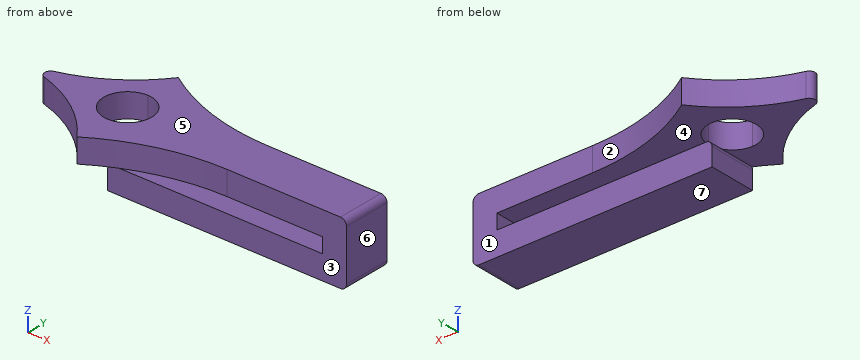
```python
from build123d import *

# Parameters (mm, degrees)
F4_DEPTH = 2
F5_DEPTH = 1.25
F6_START = -1.25
F6_DEPTH = 2
F8_DEPTH = 4


# Not quite as in the source:
# - a feature names something its author has since deleted; it is built from what else it names


with BuildPart() as f4:
    # F3 (on Top) → F4 (new body)
    with BuildSketch(Plane.XY):
        with BuildLine():
            Line((0, -2), (0, 0))
            Line((0, 0), (0, 2))
            Line((0, 2), (-8, 2))
            Line((-8, 2), (-18, 2))
            ThreePointArc((-18, 2), (-16.5857864376, 1.4142135624), (-16, 0))
            ThreePointArc((-16, 0), (-16.5857864376, -1.4142135624), (-18, -2))
            Line((-18, -2), (-8, -2))
            Line((-8, -2), (0, -2))
        make_face()
        Polygon((0, 2), (0, 0), (0, -2), (2, -2), (2, 2), align=None)
        with BuildLine():
            Line((-18, 2), (-8, 2))
            ThreePointArc((-8, 2), (-13.2201532545, 2.7661558185), (-18, 5))
            ThreePointArc((-18, 5), (-20.9134084444, 2.2029023447), (-24.5666209478, 0.4807692308))
            ThreePointArc((-24.5666209478, 0.4807692308), (-24.9292857857, 0), (-24.5666209478, -0.4807692308))
            ThreePointArc((-24.5666209478, -0.4807692308), (-20.9134084444, -2.2029023447), (-18, -5))
            ThreePointArc((-18, -5), (-13.2201532545, -2.7661558185), (-8, -2))
            Line((-8, -2), (-18, -2))
            ThreePointArc((-18, -2), (-20, 0), (-18, 2))
        make_face()
    extrude(amount=F4_DEPTH)

    # F3 (on Top) → F5 (join)
    with BuildSketch(Plane.XY):
        Polygon((0, 2), (0, 0), (0, -2), (2, -2), (2, 2), align=None)
    extrude(amount=-F5_DEPTH)

    # F3 (on Top) → F6 (join)
    with BuildSketch(Plane.XY.offset(F6_START)):
        with BuildLine():
            Line((0, -2), (0, 0))
            Line((0, 0), (0, 2))
            Line((0, 2), (-8, 2))
            Line((-8, 2), (-18, 2))
            ThreePointArc((-18, 2), (-16.5857864376, 1.4142135624), (-16, 0))
            ThreePointArc((-16, 0), (-16.5857864376, -1.4142135624), (-18, -2))
            Line((-18, -2), (-8, -2))
            Line((-8, -2), (0, -2))
        make_face()
        Polygon((0, 2), (0, 0), (0, -2), (2, -2), (2, 2), align=None)
        with BuildLine():
            ThreePointArc((-16, 0), (-16.5857864376, 1.4142135624), (-18, 2))
            Line((-18, 2), (-18, -2))
            ThreePointArc((-18, -2), (-16.5857864376, -1.4142135624), (-16, 0))
        make_face()
    extrude(amount=-F6_DEPTH)

    # F7 (on face) → F8 (cut)
    with BuildSketch(Plane.XZ.offset(2)):
        with BuildLine():
            Line((-18, -1.25), (-18, -1.75))
            ThreePointArc((-18, -1.75), (-17.8535533906, -1.3964466094), (-17.5, -1.25))
            Line((-17.5, -1.25), (-18, -1.25))
        make_face()
        with BuildLine():
            ThreePointArc((1.5, 2), (1.8535533906, 1.8535533906), (2, 1.5))
            Line((2, 1.5), (2, 2))
            Line((2, 2), (1.5, 2))
        make_face()
        with BuildLine():
            ThreePointArc((2, -2.75), (1.8535533906, -3.1035533906), (1.5, -3.25))
            Line((1.5, -3.25), (2, -3.25))
            Line((2, -3.25), (2, -2.75))
        make_face()
    extrude(amount=-F8_DEPTH, mode=Mode.SUBTRACT)


solid = f4.part
```
CAD build for the part. Positions are in the model's coordinates, mm. Face numbers are marked on the shaded views. A direction names the side the tool comes from. Round coordinates to 2 decimals unless told otherwise and drop trailing zeros. Loops run counter-clockwise (first coordinate to the right, second up) from the corner with the lowest first, then second, coordinate; pieces in that order, holes last. Notation, with made-up numbers: (9.5, 82) - (13.5, 82) arc R29 cw to (13.5, 102) - close; hole circle Ø1 at (24, 37.5). An arc over 180 degrees is marked (long way). Return JSON: item names as keys, results as strings. Group by question number.
Q1. Band-saw the part on D-D on z = -2.1. Give the cut face in (x, y), plus the area to 3 significant figures.
Q2. Band-saw the part on A-A on z = 0.9. Give the cut face in (x, y).
Q3. Two-plate mould, pull along Z, no slides. Class the marked faces 4, 5, 6 and 7: +Z half, -Z half, draft (parallel to the pull), parting line (faces both ways), or undercut.
Q4. Band-saw the part on C-C on x = -17. Give the cut face in (y, z).
Q5. Tool access for the marked faces 1, 2 and 3: list every direction of +Z, -Z, +X, -X, +Y, -Y with a clear straight run to the whole face (end or side of a thin tool).
Q6. Drill centre lines: line 1 along Z through (x, y) = (-6.5, 0.5); line 2 along Z through (x, y) = (-18.5, 4.25); line 3 along Y through (x, z) = (-2, 0.3). Where is each one in solid material? Low to high. Write a range as [from, to].
Q7. Band-saw the part on B-B on x = -9.5. Give the cut face in (y, z).
Q8. Flat gauge pins, fed straight in: pin 1 Ø2.5 at (x, z) = (-3.5, 0) entering from -Y; pin 2 Ø1.4 at (y, z) = (0, -0.5) entering from -X; pin 3 Ø0.8 at (y, z) = (0, -2.5) entering from -X. Where does each tip first touch, or does it go through?
Solutions:
{
 "1": {"outline": "(-18, -2) - (2, -2) - (2, 2) - (-18, 2) - close", "area": "80.0 mm^2"},
 "2": {"outline": "(-24.57, -0.48) arc R12.5 cw to (-18, -5) arc R18.17 cw to (-8, -2) - (2, -2) - (2, 2) - (-8, 2) arc R18.17 cw to (-18, 5) arc R12.5 cw to (-24.57, 0.48) arc R0.5 ccw to start; hole circle Ø4 at (-18, 0)"},
 "3": {"face 4": "undercut", "face 5": "+Z half", "face 6": "draft", "face 7": "-Z half"},
 "4": {"outline": "(-4.39, 0) - (-1.73, 0) - (-1.73, 2) - (-4.39, 2) - close; (-2, -3.25) - (2, -3.25) - (2, -1.25) - (-2, -1.25) - close; (1.73, 0) - (4.39, 0) - (4.39, 2) - (1.73, 2) - close"},
 "5": {"face 1": "-Z, +X, +Y", "face 2": "+Z, -Z, +X, +Y", "face 3": "-Z, +X, -Y"},
 "6": {"line 1": "z = [-3.25, -1.25], [0, 2]", "line 2": "z = [0, 2]", "line 3": "y = [-2, 2]"},
 "7": {"outline": "(-2.06, 0) - (2.06, 0) - (2.06, 2) - (-2.06, 2) - close; (-2, -3.25) - (2, -3.25) - (2, -1.25) - (-2, -1.25) - close"},
 "8": {"pin 1": "stops at y = -2", "pin 2": "stops at x = -24.93", "pin 3": "stops at x = -18"}
}
